Geometry: final body of the model. Coordinates: model frame, mm. A direction names the side the tool comes from. Round coordinates to 2 decimals unless told otherwise and drop trailing zeros. Loops run counter-clockwise (first coordinate to the right, second up) from the corner with the lowest first, then second, coordinate; pieces in that order, holes last. Notation, with made-up numbers: (76, 23.5) - (94, 23.5) arc R13 cw to (94, 31.5) - close; hole circle Ø7 at (53, -6.75). An arc over 180 degrees is marked (long way). Return JSON: item names as keys, results as strings. Group by question number.
1. Section A-A on z = -1.5. Return loops of the section in (x, y).
2. Set-up query: faces 1 (the face through (17.31, 0.2, 27.39)), 2 (the face through (0.2, 0.2, -25.4)). Return all of +Z, -Z, +X, -X, +Y, -Y with unobstructed straight access to the full face (end or side cutting, diameter ignored); none if empty.
3. First-contact query: pin 1 Ø5 at (x, z) = (-8, 24.11) entering from -Y. Flat tip, straight axial feed; report the tip coordinate or a pass-through.
4. Draft query along Z for faces 3 (the face through (-8.3, 0, -24.3)), 4 (the face through (-15.914, 0.197, -23.208)), 5 (the face through (-25.265, 0.197, -20.284)), 6 (the face through (26.68, 0.2, 3.63)). Return one class per face: +Z half, -Z half, draft (parallel to the pull), parting line (faces both ways), or undercut.
5. Section B-B on x = 0. Return loops of the section in (y, z).
6. Material intervals for probe 1 along X at (y, z) = (0.25, -23); probe 2 along X at (y, z) = (0.1, 23); probe 3 along X at (y, z) = (0.25, 26), sorted ascending.
7. Section C-C on y = 0.15. Return loops of the section in (x, z), and give its area (3 significant figures).
8. Section D-D on z = -23. Return loops of the section in (x, y), and give its area (3 significant figures).
from build123d import *

# Parameters (mm, degrees)
SKETCH1_R           = 1.6
BOSS_EXTRUDE1_DEPTH = 0.4


with BuildPart() as part:
    # Sketch1 → Boss-Extrude1 (new body)
    with BuildSketch(Plane(origin=(0, 0, 0), x_dir=(1, 0, 0), z_dir=(0, 1, 0))):
        with BuildLine():
            Line((29.237843605, 13.960963482), (24.049079653, -21.711788683))
            ThreePointArc((24.049079653, -21.711788683), (17.208573183, -27.452231403), (9.060814288, -31.107260317))
            Line((9.060814288, -31.107260317), (-9.060814288, -31.107260317))
            ThreePointArc((-9.060814288, -31.107260317), (-24.689356555, 20.980840614), (29.237843605, 13.960963482))
        make_face()
        with Locations(Location((-17.5, 23, 0), (0, 0, 270))):
            Circle(SKETCH1_R, mode=Mode.SUBTRACT)
        with Locations(Location((-17.5, -23, 0), (0, 0, 270))):
            Circle(SKETCH1_R, mode=Mode.SUBTRACT)
        with Locations(Location((17.5, -23, 0), (0, 0, 270))):
            Circle(SKETCH1_R, mode=Mode.SUBTRACT)
        with Locations(Location((17.5, 23, 0), (0, 0, 270))):
            Circle(SKETCH1_R, mode=Mode.SUBTRACT)
        with BuildLine():
            Line((-4, -24.107260317), (4, -24.107260317))
            ThreePointArc((4, -24.107260317), (8.793181532, -28.027829543), (11.685431528, -22.552398764))
            ThreePointArc((11.685431528, -22.552398764), (21.475216761, -13.563740822), (25.385385277, -0.861518628))
            ThreePointArc((25.385385277, -0.861518628), (24.952949632, 13.588699396), (13.048984262, 21.791833556))
            ThreePointArc((13.048984262, 21.791833556), (0, 25.4), (-13.048984262, 21.791833556))
            ThreePointArc((-13.048984262, 21.791833556), (-24.952949632, 13.588699396), (-25.385385277, -0.861518628))
            ThreePointArc((-25.385385277, -0.861518628), (-21.475216761, -13.563740822), (-11.685431528, -22.552398764))
            ThreePointArc((-11.685431528, -22.552398764), (-8.793181532, -28.027829543), (-4, -24.107260317))
        make_face(mode=Mode.SUBTRACT)
    extrude(amount=BOSS_EXTRUDE1_DEPTH)


solid = part.part
Taken from the geometry:
{
 "1": {"outline": "(-32.37, 0) - (-26.27, 0) - (-26.27, 0.4) - (-32.37, 0.4) - close; (26.27, 0) - (27.43, 0) - (27.43, 0.4) - (26.27, 0.4) - close"},
 "2": {"face 1": "+Z, +X, +Y, -Y", "face 2": "+Y, -Y"},
 "3": {"pin 1": "through"},
 "4": {"face 3": "draft", "face 4": "undercut", "face 5": "parting line", "face 6": "+Z half"},
 "5": {"outline": "(0, -32.4) - (0.4, -32.4) - (0.4, -25.4) - (0, -25.4) - close; (0, 24.11) - (0.4, 24.11) - (0.4, 31.11) - (0, 31.11) - close"},
 "6": {"probe 1": "-22.82 to -19.1, -15.9 to -10.78, 10.78 to 15.9, 19.1 to 22.82", "probe 2": "-22.82 to -19.1, -15.9 to -11.84, 11.84 to 15.9, 19.1 to 22.82", "probe 3": "-19.33 to -11.52, -4.48 to 4.48, 11.52 to 19.33"},
 "7": {"outline": "(-9.06, 31.11) arc R32.4 ccw (long way) to (29.24, -13.96) - (24.05, 21.71) arc R32.4 ccw to (9.06, 31.11) - close; hole (-25.39, 0.86) arc R16 ccw to (-13.05, -21.79) arc R25.4 ccw to (13.05, -21.79) arc R16 ccw to (25.39, 0.86) arc R25.4 ccw to (11.69, 22.55) arc R4 ccw (long way) to (4, 24.11) - (-4, 24.11) arc R4 ccw (long way) to (-11.69, 22.55) arc R25.4 ccw to start; hole circle Ø3.2 at (-17.5, -23); hole circle Ø3.2 at (-17.5, 23); hole circle Ø3.2 at (17.5, -23); hole circle Ø3.2 at (17.5, 23)", "area": "934 mm2"},
 "8": {"outline": "(-22.82, 0) - (-19.1, 0) - (-19.1, 0.4) - (-22.82, 0.4) - close; (-15.9, 0) - (-10.78, 0) - (-10.78, 0.4) - (-15.9, 0.4) - close; (10.78, 0) - (15.9, 0) - (15.9, 0.4) - (10.78, 0.4) - close; (19.1, 0) - (22.82, 0) - (22.82, 0.4) - (19.1, 0.4) - close", "area": "7.07 mm2"}
}
